Build history of the part. All positions in model axes, mm. Face numbers are marked on the shaded views. A direction names the side the tool comes from. Round coordinates to 2 decimals unless told otherwise and drop trailing zeros. Write each loop counter-clockwise with the first axis right and the second up, starting at its lowest first coordinate (ties: lowest second). Pieces come first, ordered by that corner, then holes.
1) Which spindle directions (+Z, -Z, +X, -X, +Y, -Y) get a long thin tool onto all of the face, cutting with end or side? Do the marked faces 1, 2 and 3. Say none if no direction does.
2) Saw through at C-C (y = -4). Write the cut outline in (x, z).
3) Flat gauge pins, fed straight in: pin 1 (2.5 mm diameter, centred on x = 1, z = -1, fed in from -Y); pin 2 (1.5 mm diameter, centred on x = 1.5, y = -4, fed in from +Z). Where does each tip first touch, or does it go through?
4) Saw through at B-B (z = 0). Write the cut outline in (x, y), plus the area to 3 significant figures.
5) Saw through at D-D (z = -2.2). Write the cut outline in (x, y), plus the area to 3 significant figures.
6) Wall check: probe 1 along Y at (x, z) = (-1.15, 1.85); probe 2 along Z at (x, y) = (-0.05, -2.25); probe 3 along X at (y, z) = (-2.75, -0.1). Give the ranges that are in metal, low to high.
7) Saw through at A-A (x = 0). Write the cut outline in (y, z).
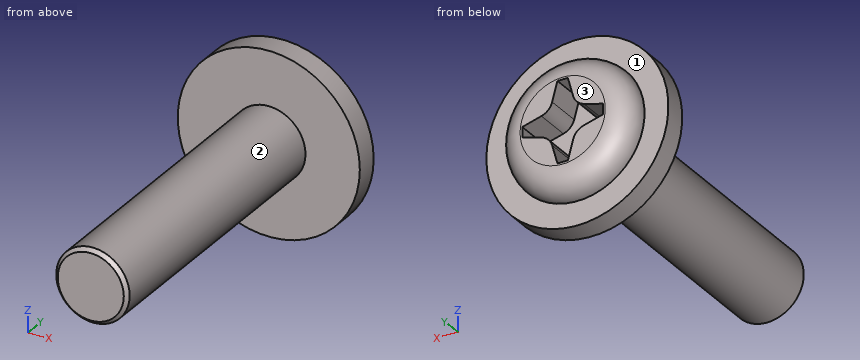
from build123d import *

# Parameters (mm, degrees)
CUT_EXTRUDE1_DEPTH = 1


with BuildPart() as part:
    # Sketch1 → Revolve1 (revolve)
    with BuildSketch(Plane.XY):
        with BuildLine():
            Line((0, -9.4), (0.9, -9.4))
            Line((0.9, -9.4), (1, -9.3))
            Line((1, -9.3), (1, -1.3))
            Line((1, -1.3), (2.48, -1.3))
            Line((2.48, -1.3), (2.48, -0.67))
            Line((2.48, -0.67), (1.83, -0.67))
            ThreePointArc((1.83, -0.67), (1.633761543, -0.196238457), (1.16, 0))
            Line((1.16, 0), (0, 0))
            Line((0, 0), (0, -9.4))
        make_face()
    revolve(axis=Axis((0, 0, 0), (0, -1, 0)))

    # Sketch2 → Cut-Extrude1 (cut)
    with BuildSketch(Plane(origin=(0, 0, 0), x_dir=(1, 0, 0), z_dir=(0, 1, 0))):
        with BuildLine():
            Line((0, 1.1), (0.141406897, 1.1))
            Line((0.141406897, 1.1), (0.285471459, 0.578570854))
            ThreePointArc((0.285471459, 0.578570854), (0.393362387, 0.393362387), (0.578570854, 0.285471459))
            Line((0.578570854, 0.285471459), (1.1, 0.141406897))
            Line((1.1, 0.141406897), (1.1, 0))
            Line((1.1, 0), (1.1, -0.141406897))
            Line((1.1, -0.141406897), (0.578570854, -0.285471459))
            ThreePointArc((0.578570854, -0.285471459), (0.393362387, -0.393362387), (0.285471459, -0.578570854))
            Line((0.285471459, -0.578570854), (0.141406897, -1.1))
            Line((0.141406897, -1.1), (0, -1.1))
            Line((0, -1.1), (-0.141406897, -1.1))
            Line((-0.141406897, -1.1), (-0.285471459, -0.578570854))
            ThreePointArc((-0.285471459, -0.578570854), (-0.393362387, -0.393362387), (-0.578570854, -0.285471459))
            Line((-0.578570854, -0.285471459), (-1.1, -0.141406897))
            Line((-1.1, -0.141406897), (-1.1, 0))
            Line((-1.1, 0), (-1.1, 0.141406897))
            Line((-1.1, 0.141406897), (-0.578570854, 0.285471459))
            ThreePointArc((-0.578570854, 0.285471459), (-0.393362387, 0.393362387), (-0.285471459, 0.578570854))
            Line((-0.285471459, 0.578570854), (-0.141406897, 1.1))
            Line((-0.141406897, 1.1), (0, 1.1))
        make_face()
    extrude(amount=-CUT_EXTRUDE1_DEPTH, mode=Mode.SUBTRACT)


solid = part.part
Evaluation:
1. face 1: +Y
1. face 2: -Y
1. face 3: +Z, -Z, +X, -X, +Y
2. outline: circle Ø2 at (0, 0)
3. pin 1: stops at y = -9.4
3. pin 2: stops at z = 0.66
4. outline: (-2.48, -1.3) - (-1, -1.3) - (-1, -9.3) - (-0.9, -9.4) - (0.9, -9.4) - (1, -9.3) - (1, -1.3) - (2.48, -1.3) - (2.48, -0.67) - (1.83, -0.67) arc R0.67 ccw to (1.16, 0) - (1.1, 0) - (1.1, -1) - (-1.1, -1) - (-1.1, 0) - (-1.16, 0) arc R0.67 ccw to (-1.83, -0.67) - (-2.48, -0.67) - close
4. area: 19.4 mm2
5. outline: (-1.14, -1.3) - (1.14, -1.3) - (1.14, -0.67) - (-1.14, -0.67) - close
5. area: 1.44 mm2
6. probe 1: y = -1.3 to -0.67
6. probe 2: z = -1 to 1
6. probe 3: x = -0.99 to 0.99
7. outline: (-9.4, -0.9) - (-9.3, -1) - (-1.3, -1) - (-1.3, -2.48) - (-0.67, -2.48) - (-0.67, -1.83) arc R0.67 ccw to (0, -1.16) - (0, -1.1) - (-1, -1.1) - (-1, 1.1) - (0, 1.1) - (0, 1.16) arc R0.67 ccw to (-0.67, 1.83) - (-0.67, 2.48) - (-1.3, 2.48) - (-1.3, 1) - (-9.3, 1) - (-9.4, 0.9) - close
